Autodesk Inventor part; units mm, degrees
ref_plane "YZ Plane" through (0, 0, 0) normal (1, 0, 0) x (0, 1, 0)
ref_plane "XZ Plane" through (0, 0, 0) normal (0, 1, 0) x (-1, 0, 0)
ref_plane "XY Plane" through (0, 0, 0) normal (0, 0, 1) x (1, 0, 0)
sketch "Sketch1" plane through (0, 0, 0) normal (0, 0, 1) x (1, 0, 0)
  line L0 (-10, 5) -> (10, 5)
  line L1 (10, 5) -> (10, -5)
  line L2 (10, -5) -> (-10, -5)
  line L3 (-10, -5) -> (-10, 5)
  point P0 (0, 0)
  dimension "d0" = 20
  dimension "d1" = 10
  dimension "d2" = 5
  dimension "d3" = 10
extrude "Extrusion1" add sketch "Sketch1" along normal blind 0.5
sketch "Sketch2" plane through (0, 0, 0) normal (0, 0, -1) x (-1, 0, 0)
  circle A0 centre (9.4, 4.4) radius 0.3
  circle A1 centre (-9.4, 4.4) radius 0.3
  circle A2 centre (-9.4, -4.4) radius 0.3
  circle A3 centre (9.4, -4.4) radius 0.3
  line L0 (10, 5) -> (-10, 5)
  line L1 (-10, 5) -> (-10, -5)
  line L2 (10, -5) -> (10, 5)
  line L3 (-10, -5) -> (10, -5)
  point P0 (0, 0)
  dimension "d6" = 0.6
  dimension "d7" = 0.6
  dimension "d8" = 0.6
  dimension "d9" = 0.6
  dimension "d10" = 0.6
  dimension "d11" = 0.6
  dimension "d12" = 0.6
  dimension "d13" = 0.6
  dimension "d14" = 0.6
  dimension "d15" = 0.6
  dimension "d16" = 0.6
  dimension "d17" = 0.6
extrude "Extrusion2" add sketch "Sketch2" along normal blind 7 contours A0 | A1 | A2 | A3
equation "\"d1\" = 0.5 * d0"
equation "\"d7\" = d6"
equation "\"d8\" = d7"
equation "\"d9\" = d7"
equation "\"d10\" = d6"
equation "\"d11\" = d8"
equation "\"d12\" = d6"
equation "\"d13\" = d7"
equation "\"d14\" = d8"
equation "\"d15\" = d6"
equation "\"d16\" = d7"
equation "\"d17\" = d8"
properties part number "PythonKukaTable"
Geometry check sheet. Reference: the model listing, model coordinates, mm. Round coordinates to 2 decimals unless told otherwise and drop trailing zeros. Loops run counter-clockwise (first coordinate to the right, second up) from the corner with the lowest first, then second, coordinate; pieces in that order, holes last. Notation, with made-up numbers: (-11.75, 5) -> (-0.75, 5) arc R25 cw to (-0.75, 37) -> close; hole circle Ø7 at (-17, 18.5). An arc over 180 degrees is marked (long way). Answer as a JSON object with one key per item and string values. Group by question number.
Item 1: Cross-section at C-C, the plane y = -4.4. Record the cut outline in (x, z).
Item 2: Depth check by flat-ended pin: pin 1 Ø2 at (x, y) = (6, -1.5) entering from -Z; pin 2 Ø1.5 at (y, z) = (3, -5.5) entering from +X. Enter the tip coordinate at first touch or a pass-through.
Item 3: Cross-section at A-A, the plane x = -9.4. Record the cut outline in (y, z).
Item 4: Thickness scan on line 1 along Z through (x, y) = (-2.5, 3.25). Record the ranges inside material, lowest first.
Item 5: Cross-section at B-B, the plane z = -4.75. Record the cut outline in (x, y).
Item 6: Cross-section at D-D, the plane y = 0. Record the cut outline in (x, z), plus the area to 3 significant figures.
Determined:
{
 "1": {"outline": "(-10, 0) -> (-9.7, 0) -> (-9.7, -7) -> (-9.1, -7) -> (-9.1, 0) -> (9.1, 0) -> (9.1, -7) -> (9.7, -7) -> (9.7, 0) -> (10, 0) -> (10, 0.5) -> (-10, 0.5) -> close"},
 "2": {"pin 1": "stops at z = 0", "pin 2": "passes through"},
 "3": {"outline": "(-5, 0) -> (-4.7, 0) -> (-4.7, -7) -> (-4.1, -7) -> (-4.1, 0) -> (4.1, 0) -> (4.1, -7) -> (4.7, -7) -> (4.7, 0) -> (5, 0) -> (5, 0.5) -> (-5, 0.5) -> close"},
 "4": {"line 1": "z = 0 to 0.5"},
 "5": {"outline": "circle Ø0.6 at (-9.4, -4.4); circle Ø0.6 at (-9.4, 4.4); circle Ø0.6 at (9.4, -4.4); circle Ø0.6 at (9.4, 4.4)"},
 "6": {"outline": "(-10, 0) -> (10, 0) -> (10, 0.5) -> (-10, 0.5) -> close", "area": "10.0 mm²"}
}
